Input: part model. Units: mm. Frame: model coordinates. Face numbers are marked on the shaded views. A direction names the side the tool comes from. Coordinates: 2 decimals unless noted, no trailing zeros. Loops run counter-clockwise (first coordinate to the right, second up) from the corner with the lowest first, then second, coordinate; pieces in that order, holes last. Notation, with made-up numbers: (-32.75, 40.25) -> (-23.75, 40.25) arc R25 ccw to (-23.75, 64.25) -> close; hole circle Ø2 at (-0.5, -7.5). An arc over 180 degrees is marked (long way). Put each result on its own line as item: value. Start each with the question number.
1) Material intervals for L1, parallel to X at y = -29.5, z = 36.5; L2, parallel to Z at x = 34.5, y = 24; L3, parallel to Y at x = 11, z = 20, sorted ascending.
2) Cut plane B-B (x = 28). Return the cut outline in (y, z).
3) Set-up query: the marked faces 1, 2 and 3. Return all of +Z, -Z, +X, -X, +Y, -Y with unobstructed straight access to the full face (end or side cutting, diameter ignored); none if empty.
4) Cut plane C-C (y = -4.5). Return the cut outline in (x, z).
5) Cut plane A-A (z = 39.5). Return the cut outline in (x, y).
6) Cut plane D-D (z = 20). Return the cut outline in (x, y).
7) Pull-direction query (Z, two-part tool) for the marked faces 4, 5 and 6; classes: pulls with the +Z half, pulls with the -Z half, needs draft (parallel to the pull), parting line crosses it, or undercut.
8) Contact query for flat-ended pins moving along their axis: P1, Ø5, axis at y = -28, z = 31, coming from the +X side; P2, Ø16.5, axis at x = 48.5, y = -26.5, coming from the +Z side; P3, Ø12, axis at y = -26, z = 27, coming from the -X side. Output: stop coordinate, or through.
from build123d import *

# Parameters (mm, degrees)
F0_W     = 200
F0_H     = 100
F1_DEPTH = 15
F4_DEPTH = 15
F5_W     = 30
F5_H     = 15
F6_DEPTH = 15
F7_R     = 10


with BuildPart() as f1:
    # F0 (on Top) → F1 (new body)
    with BuildSketch(Plane.XY):
        Rectangle(F0_W, F0_H)
    extrude(amount=F1_DEPTH)

    # F3 (on offset) → F4 (join)
    with BuildSketch(Plane.XZ.offset(35)):
        Polygon((10, 15), (85, 15), (85, 65), (10, 45), align=None)
    extrude(amount=-F4_DEPTH)

    # F5 (on face) → F6 (cut, through all)
    with BuildSketch(Plane.XZ.offset(35)):
        with Locations((55, 37.5)):
            Rectangle(F5_W, F5_H)
    extrude(amount=-F6_DEPTH, mode=Mode.SUBTRACT)

    # F7
    f7_edges = [f1.edges().sort_by_distance(p)[0] for p in [
        (10, -27.5, 45),
        (85, -27.5, 65),
        (100, -50, 7.5),
        (-100, -50, 7.5),
        (-100, 50, 7.5),
        (100, 50, 7.5),
    ]]
    fillet(f7_edges, radius=F7_R)


solid = f1.part
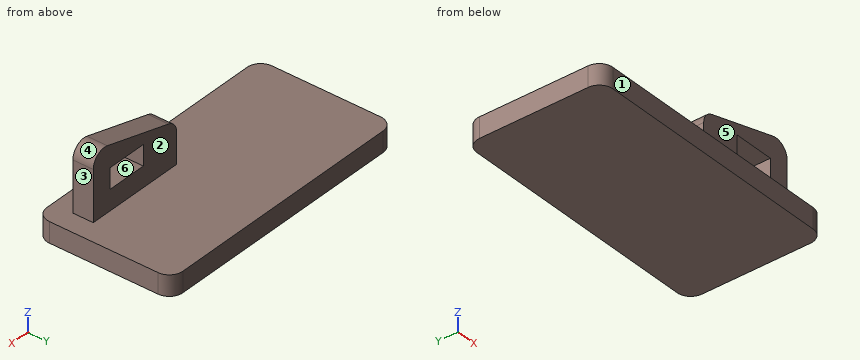
Results found:
1. L1: x = 10 to 40, 70 to 85
1. L2: z = 0 to 15
1. L3: y = -35 to -20
2. outline: (-50, 0) -> (50, 0) -> (50, 15) -> (-20, 15) -> (-20, 49.8) -> (-35, 49.8) -> (-35, 15) -> (-50, 15) -> close
3. face 1: +Z, -Z, +X, -X, -Y
3. face 2: +Z, +X, -X, +Y
3. face 3: +Z, +X, +Y, -Y
4. outline: (-100, 0) -> (100, 0) -> (100, 15) -> (-100, 15) -> close
5. outline: (10.24, -35) -> (40, -35) -> (40, -20) -> (10.24, -20) -> close; (70, -35) -> (85, -35) -> (85, -20) -> (70, -20) -> close
6. outline: (10, -35) -> (85, -35) -> (85, -20) -> (10, -20) -> close
7. face 4: pulls with the +Z half
7. face 5: needs draft
7. face 6: undercut
8. P1: stops at x = 85
8. P2: stops at z = 57.47
8. P3: stops at x = 10
